from build123d import *

# Parameters (mm, degrees)
FILLET7_R             = 2
FILLET8_R             = 2
SKETCH2_R             = 17.932362589
SKETCH2_R_2           = 4.070139316
SKETCH2_R_3           = 1.470244109
BOSS_EXTRUDE4_DEPTH   = 2
F_1_0MM_DOWEL_HOLE1_D = 1
F_1_0MM_DOWEL_HOLE3_D = 1


with BuildPart() as part:
    # Sketch1 → Revolve2 (revolve)
    with BuildSketch(Plane.XY, mode=Mode.PRIVATE) as revolve2_sk:
        Polygon((-22.5, 0), (22.5, 0), (22.5, 5), (22.5, 10), (12.5, 10), (12.5, 5), (-17.5, 5), (-17.5, 20), (-22.5, 20), align=None)
    revolve(revolve2_sk.sketch.rotate(Axis((-22.5, 0, 0), (1, 0, 0)), 90), axis=Axis((-22.5, 0, 0), (1, 0, 0)))

    # Fillet7
    fillet7_edges = [part.edges().sort_by_distance(p)[0] for p in [
        (22.5, 0, -10),
    ]]
    fillet(fillet7_edges, radius=FILLET7_R)

    # Fillet8
    fillet8_edges = [part.edges().sort_by_distance(p)[0] for p in [
        (12.5, 0, -10),
    ]]
    fillet(fillet8_edges, radius=FILLET8_R)

    # Sketch2 → Boss-Extrude4 (add)
    # profile 1 of 7: a face of its own
    with BuildSketch(Plane.ZY.offset(22.5)):
        Polygon((0, 20), (-14.142135624, 14.142135624), (-20, 0), (-14.142135624, -14.142135624), (0, -20), (14.142135624, -14.142135624), (20, 0), (14.142135624, 14.142135624), align=None)
        Circle(SKETCH2_R, mode=Mode.SUBTRACT)
    # profile 2 of 7: a face of its own
    with BuildSketch(Plane.ZY.offset(22.5)):
        with Locations((7.5, 6.359605711)):
            Circle(SKETCH2_R_2)
        with Locations((7.5, 6.359605711)):
            Circle(SKETCH2_R_3, mode=Mode.SUBTRACT)
    # profile 3 of 7: a face of its own
    with BuildSketch(Plane.ZY.offset(22.5)):
        with Locations((-7.5, 6.816829323)):
            Circle(SKETCH2_R_2)
        with Locations((-7.5, 6.816829323)):
            Circle(SKETCH2_R_3, mode=Mode.SUBTRACT)
    # profile 4 of 7: a face of its own
    with BuildSketch(Plane.ZY.offset(22.5)):
        Polygon((-5.383481764, 14.709120363), (-1.33333, 10.377946656), (-3.850746579, 9.493506516), (-6.434561549, 12.256600867), align=None)
    # profile 5 of 7: a face of its own
    with BuildSketch(Plane.ZY.offset(22.5)):
        with BuildLine():
            Line((-11.570139316, -4.68431352), (11.757283774, -4.68431352))
            add(Edge.make_bspline(
                [(-11.570139316, -4.68431352), (0.019330621, -23.600400847), (11.757283774, -4.68431352)],
                knots=[0, 0, 0, 1, 1, 1], degree=2))
        make_face()
        with BuildLine():
            Line((-7.5, -6.493557604), (7.5, -6.493557604))
            add(Edge.make_bspline(
                [(7.5, -6.493557604), (0, -19.67127169), (-7.5, -6.493557604)],
                knots=[0, 0, 0, 1, 1, 1], degree=2))
        make_face(mode=Mode.SUBTRACT)
    # profile 6 of 7: a face of its own
    with BuildSketch(Plane.ZY.offset(22.5)):
        Polygon((5.664503708, 14.42809842), (1.33333, 10.377946656), (3.785849496, 9.326866872), (6.548943848, 11.910681841), align=None)
    # profile 7 of 7: a face of its own
    with BuildSketch(Plane.ZY.offset(22.5)):
        Polygon((-0.404292244, 2.684485233), (2.559752906, -0.834695524), (-2.116560108, -1.19469663), align=None)
    extrude(amount=BOSS_EXTRUDE4_DEPTH)

    # Ø1.0mm Dowel Hole1 (through all)
    with Locations(Plane(origin=(22.5, 0, 0), x_dir=(0, 0, -1), z_dir=(1, 0, 0))):
        with Locations((1.693680894, 1.577447892)):
            Hole(F_1_0MM_DOWEL_HOLE1_D / 2)

    # Ø1.0mm Dowel Hole3 (through all)
    with Locations(Plane.ZY.offset(22.5)):
        with Locations((15.708060058, 0), (-15.575222341, 0), (0, -16.687738223)):
            Hole(F_1_0MM_DOWEL_HOLE3_D / 2)


solid = part.part
Could you check a few things on this model? Use its own coordinates, in mm. A direction names the side the tool comes from. Give positions to 0.01 mm unless a question says otherwise; leave off trailing zeros. Order: outer loops, then holes, each group sorted by start corner. A loop starts at its lowest first (then second) coordinate and runs counter-clockwise, first axis right, second up.
Item 1: I'm going to push flat-ended pins straight in: pin 1 (4.5 mm diameter, centred on y = 5, z = -16.5, fed in from -X); pin 2 (2 mm diameter, centred on x = -24, z = 5.5, fed in from +Y); pin 3 (10 mm diameter, centred on x = 7, z = 5.5, fed in from -Y); pin 4 (1 mm diameter, centred on y = 7, z = 14, fed in from +X). Where does each tip first touch, or does it pass through?
Item 2: If we section it at C-C, the plane x = -11: Write out the boundary of the cut face in (y, z), plus the area to 3 significant figures.
Item 3: If we section it at A-A, the plane x = -21.5: Write out the boundary of the cut face in (y, z), plus the area to 3 significant figures.
Item 4: For faces 1 (the face through (-24.5, 6.4, 9.3)), 2 (the face through (-23.5, 0.9, 1.1)), 3 (the face through (-22.5, 7, -18)), 4 (the face through (-22.5, 17.5, 7)), 5 (the face through (-22.5, -7, 18)), which set-ups out of +Z, -Z, +X, -X, +Y, -Y let a thin tool reach every point of the face, with its end or its side?
Item 5: If we section it at B-B, the plane z = -12.5: Write out the boundary of the cut face in (x, y), plus the area to 3 significant figures.
Item 6: If we mould it in two halves opening along Y, with no side actions, what happens to faces 6 (the face through (-22.5, 6, 7)), 7 (the face through (-22.5, -18, 7)), 8 (the face through (-23.49, 0.72, -1.27)), 9 (the face through (-23.49, 17.03, 7.17))? For each: pulls with the +Y half, pulls with the -Y half, needs draft (parallel to the pull), parting line crosses it, or undercut.
Item 7: I need wall thicknesses on line 1 (Y direction, x = -23, z = -7); line 2 (X direction, y = -7, z = 2); line 3 (X direction, y = -5, z = 2). Which ranges of each line are inside material? Lowest first, please.
Values:
1. pin 1: stops at x = -24.5
1. pin 2: stops at y = 18.14
1. pin 3: stops at y = -4.97
1. pin 4: stops at x = -17.5
2. outline: circle Ø10 at (0, 0); hole circle Ø1 at (1.58, -1.69)
2. area: 77.8 mm2
3. outline: circle Ø40 at (0, 0); hole circle Ø1 at (-16.69, 0); hole circle Ø1 at (0, -15.58); hole circle Ø1 at (0, 15.71); hole circle Ø1 at (1.58, -1.69)
3. area: 1,250 mm2
4. face 1: +Z, -Z, -X, +Y, -Y
4. face 2: -X
4. face 3: -Z, -X, +Y
4. face 4: +Z, -X, +Y
4. face 5: +Z, -X, -Y
5. outline: (-24.5, -14.82) - (-22.5, -14.82) - (-22.5, -15.61) - (-17.5, -15.61) - (-17.5, 15.61) - (-22.5, 15.61) - (-22.5, 14.82) - (-24.5, 14.82) - (-24.5, 12.86) - (-22.5, 12.86) - (-22.5, -12.86) - (-24.5, -12.86) - close
5. area: 164 mm2
6. face 6: undercut
6. face 7: needs draft
6. face 8: undercut
6. face 9: pulls with the +Y half
7. line 1: y = -17.1 to -16.51, -10.67 to -7.34, -6.49 to -4.68, 2.78 to 5.43, 8.2 to 10.86, 16.51 to 17.1
7. line 2: x = -22.5 to -17.5, 12.5 to 22.5
7. line 3: x = -24.5 to -17.5, 12.5 to 22.5
